Check sheet for the modelled part. Datum: model origin and axes. Units: mm. Round coordinates to 2 decimals unless told otherwise and drop trailing zeros. Write each loop counter-clockwise with the first axis right and the second up, starting at its lowest first coordinate (ties: lowest second). Pieces come first, ordered by that corner, then holes. Notation, with made-up numbers: (51.25, -14.75) -> (77.25, -14.75) arc R32 ccw to (77.25, 17.25) -> close; hole circle Ø6 at (-16, 60.5). An arc over 180 degrees is marked (long way). One line per item, written item: value.
from build123d import *

# Parameters (mm, degrees)
F1_DEPTH = 6.35
F2_SIZE  = 6.34999
F3_SIZE2 = 6.0705106322
F3_SIZE  = 55.88


# Not quite as in the source:
# - a fillet or chamfer is up to 0.001 mm smaller than in the source, because OpenCascade refuses the exact size


with BuildPart() as f1:
    # F0 (on Top) → F1 (new body)
    with BuildSketch(Plane.XY):
        Polygon((75, 225), (-75, 225), (-29.020415619, 152.489066124), (29.020415619, 152.489066124), align=None)
    extrude(amount=F1_DEPTH)

    # F2 (size 6.35 in the source; OpenCascade refuses exactly that, so slightly less here)
    f2_edges = [f1.edges().sort_by_distance(p)[0] for p in [
        (0, 225, 0),
    ]]
    chamfer(f2_edges, length=F2_SIZE)

    # F3
    f3_edges = [f1.edges().sort_by_distance(p)[0] for p in [
        (0, 152.489066, 6.35),
    ]]
    f3_side = f1.faces().sort_by_distance((0, 194.086469, 6.35))[0]
    chamfer(f3_edges, length=F3_SIZE, length2=F3_SIZE2, reference=f3_side)


solid = f1.part
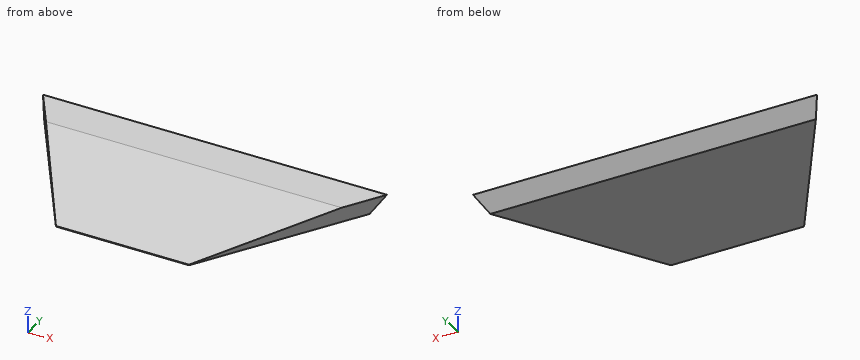
Item 1: Material ranges on line 1 along X through (y, z) = (194, 2); line 2 along Y through (x, z) = (51, 3); line 3 along Y through (x, z) = (58, 4.25), recorded low to high.
Result set:
line 1: -55.34 to 55.34
line 2: 187.15 to 221.65
line 3: 198.19 to 222.9
Item 2: Sectioned sample at B-B (z = 4.5). Enter the section's corners in (x, y).
Result set:
outline: (-73.83, 223.15) -> (-53.66, 191.34) -> (53.66, 191.34) -> (73.83, 223.15) -> close
Item 3: Depth check by flat-ended pin: pin 1 (2 mm diameter, centred on x = 37.5, z = 2, fed in from -Y); pin 2 (1 mm diameter, centred on x = 7, z = 2, fed in from +Y); pin 3 (1.5 mm diameter, centred on y = 198, z = 2.5, fed in from +X). Enter the tip coordinate at first touch or a pass-through.
Result set:
pin 1: y = 164.43
pin 2: y = 221.15
pin 3: x = 58.35
Item 4: Sectioned sample at C-C (y = 192.5). Enter the section's corners in (x, z).
Result set:
outline: (-54.39, 0) -> (54.39, 0) -> (54.39, 4.63) -> (-54.39, 4.63) -> close
